Can you work these out from the model? Positions are in its coordinate system, mm. Face numbers are marked on the shaded views. A direction names the side the tool comes from. Give positions to 0.01 mm unless a question says otherwise; leave off trailing zeros. Order: outer loops, then holes, each group sorted by start corner. A loop starts at its lowest first (then second) coordinate and runs counter-clockwise, first axis right, second up. Notation, with made-up numbers: (83, 50) - (116, 50) arc R17 cw to (116, 76) - close; hole circle Ø5 at (2.25, 39.25). An arc over 180 degrees is marked (long way). Use one line per item in the form item = value. Start each with the question number.
1) Suppose I cut it at A-A, the plane y = 36. Write out the boundary of the cut face in (x, z), and give its area (3 significant figures).
2) Suppose I cut it at D-D, the plane y = 0. Write out the boundary of the cut face in (x, z), and give its area (3 significant figures).
3) Please list where these lines run through material, in increasing order: probe 1 along Z at (x, y) = (9.4, 0); probe 2 along Z at (x, y) = (-62, -10); probe 3 along X at (y, z) = (-7, 68.5).
4) Suppose I cut it at B-B, the plane x = -11. Write out the boundary of the cut face in (y, z).
5) Suppose I cut it at C-C, the plane z = 32. Write out the boundary of the cut face in (x, y), and give its area (3 significant figures).
6) Which directions (+Z, -Z, +X, -X, +Y, -Y) give clear straight access to the entire face, cutting with the end or side of a thin tool? Please do the marked faces 1, 2, 3, 4 and 5.
7) For pin 1 (12 mm diameter, centred on y = 65.5, z = 15.5, fed in from +X); pin 2 (9 mm diameter, centred on y = -6.5, z = 113.5, fed in from -X); pin 3 (1 mm diameter, centred on y = 22, z = 72, fed in from +X); pin 4 (12 mm diameter, centred on x = -35.5, y = 19, fed in from +Z), each with a flat end and sliding along its axis, tell me the tip position at first contact or that it passes through.
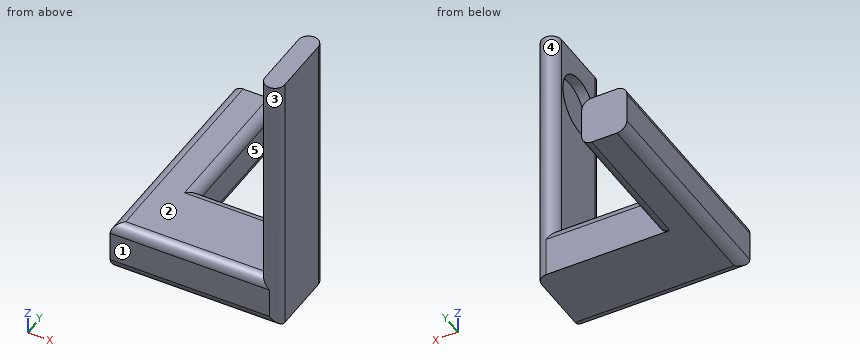
```python
from build123d import *

# Parameters (mm, degrees)
F0_W         = 70
F0_H         = 40
F0_W_2       = 15
F1_DEPTH     = 25
F2_W         = 10
F2_H         = 40
F3_DEPTH     = 110
F4_W         = 22.7000065148
F4_H         = 25
F5_DEPTH     = 70
F6_R         = 14.75
F7_DEPTH     = 5
F8_T1_DEPTH  = 87.5
F8_T3_DEPTH  = 52.2999934852
F8_T5_DEPTH  = 82.5
F8_T7_DEPTH  = 135
F8_T9_DEPTH  = 110
F8_T11_DEPTH = 160
F8_T13_DEPTH = 122.5
F8_T19_DEPTH = 100
F8_T23_DEPTH = 135
F8_T30_DEPTH = 64.7999934852
F8_T34_DEPTH = 135
F8_T41_DEPTH = 64.7999934852
F8_T45_DEPTH = 95


# Not quite as in the source:
# - a fillet or chamfer that OpenCascade refuses, or shapes differently, is made with other operations: its cross-section is extruded or revolved along the edge and cut away or added


with BuildPart() as f1:
    # F0 (on Top) → F1 (new body)
    with BuildSketch(Plane.XY):
        with Locations((-33.8003174961, 0.9457613719)):
            Rectangle(F0_W, F0_H)
        with Locations((8.6996825039, 0.9457613719)):
            Rectangle(F0_W_2, F0_H)
    extrude(amount=F1_DEPTH)

    # F2 (on face) → F3 (join)
    with BuildSketch(Plane.XY.offset(25)):
        with Locations((11.1996825039, 0.9457613719)):
            Rectangle(F2_W, F2_H)
    extrude(amount=F3_DEPTH)

    # F4 (on face) → F5 (join)
    with BuildSketch(Plane(origin=(0, 20.9457613719, 0), x_dir=(-1, 0, 0), z_dir=(0, 1, 0))):
        with Locations((57.4503142387, 12.5)):
            Rectangle(F4_W, F4_H)
    extrude(amount=F5_DEPTH)

    # F6 (on face) → F7 (cut)
    with BuildSketch(Plane(origin=(6.1996825039, 0, 0), x_dir=(0, -1, 0), z_dir=(-1, 0, 0))):
        with Locations((0, 108.7849736214)):
            Circle(F6_R)
    extrude(amount=-F7_DEPTH, mode=Mode.SUBTRACT)

    # F8: fillet of radius 5 on 11 edges, made by hand

    # F8_s2 → F8_t1 (cut)
    with BuildSketch(Plane.YZ.offset(-81.3003174961)):
        with BuildLine():
            ThreePointArc((-19.0542386281, 20), (-17.589772534, 23.5355339059), (-14.0542386281, 25))
            Line((-14.0542386281, 25), (-19.0542386281, 25))
            Line((-19.0542386281, 25), (-19.0542386281, 20))
        make_face()
    extrude(amount=F8_T1_DEPTH, mode=Mode.SUBTRACT)

    # F8_s4 → F8_t3 (cut)
    with BuildSketch(Plane.YZ.offset(-46.1003109813)):
        with BuildLine():
            ThreePointArc((15.9457613719, 25), (19.4812952778, 23.5355339059), (20.9457613719, 20))
            Line((20.9457613719, 20), (20.9457613719, 25))
            Line((20.9457613719, 25), (15.9457613719, 25))
        make_face()
    extrude(amount=F8_T3_DEPTH, mode=Mode.SUBTRACT)

    # F8_s6 → F8_t5 (cut)
    with BuildSketch(Plane.XZ.offset(-103.4457613719)):
        with BuildLine():
            ThreePointArc((-51.1003109813, 25), (-47.5647770753, 23.5355339059), (-46.1003109813, 20))
            Line((-46.1003109813, 20), (-46.1003109813, 25))
            Line((-46.1003109813, 25), (-51.1003109813, 25))
        make_face()
        with BuildLine():
            ThreePointArc((-51.1003109813, 0), (-47.5647770753, 1.4644660941), (-46.1003109813, 5))
            Line((-46.1003109813, 5), (-46.1003109813, 0))
            Line((-46.1003109813, 0), (-51.1003109813, 0))
        make_face()
    extrude(amount=F8_T5_DEPTH, mode=Mode.SUBTRACT)

    # F8_s8 → F8_t7 (cut)
    with BuildSketch(Plane.XZ.offset(-103.4457613719)):
        with BuildLine():
            ThreePointArc((-68.8003174961, 20), (-67.335851402, 23.5355339059), (-63.8003174961, 25))
            Line((-63.8003174961, 25), (-68.8003174961, 25))
            Line((-68.8003174961, 25), (-68.8003174961, 20))
        make_face()
        with BuildLine():
            ThreePointArc((-68.8003174961, 5), (-67.335851402, 1.4644660941), (-63.8003174961, 0))
            Line((-63.8003174961, 0), (-68.8003174961, 0))
            Line((-68.8003174961, 0), (-68.8003174961, 5))
        make_face()
    extrude(amount=F8_T7_DEPTH, mode=Mode.SUBTRACT)

    # F8_s10 → F8_t9 (cut)
    with BuildSketch(Plane.YZ.offset(-81.3003174961)):
        with BuildLine():
            ThreePointArc((-19.0542386281, 5), (-17.589772534, 1.4644660941), (-14.0542386281, 0))
            Line((-14.0542386281, 0), (-19.0542386281, 0))
            Line((-19.0542386281, 0), (-19.0542386281, 5))
        make_face()
    extrude(amount=F8_T9_DEPTH, mode=Mode.SUBTRACT)

    # F8_s12 → F8_t11 (cut)
    with BuildSketch(Plane.XY.offset(-12.5)):
        with BuildLine():
            ThreePointArc((11.1996825039, -19.0542386281), (14.7352164099, -17.589772534), (16.1996825039, -14.0542386281))
            Line((16.1996825039, -14.0542386281), (16.1996825039, -19.0542386281))
            Line((16.1996825039, -19.0542386281), (11.1996825039, -19.0542386281))
        make_face()
        with BuildLine():
            ThreePointArc((16.1996825039, 15.9457613719), (14.7352164099, 19.4812952778), (11.1996825039, 20.9457613719))
            Line((11.1996825039, 20.9457613719), (16.1996825039, 20.9457613719))
            Line((16.1996825039, 20.9457613719), (16.1996825039, 15.9457613719))
        make_face()
    extrude(amount=F8_T11_DEPTH, mode=Mode.SUBTRACT)

    # F8_s14 → F8_t13 (cut)
    with BuildSketch(Plane.XY.offset(25)):
        with BuildLine():
            ThreePointArc((11.1996825039, -19.0542386281), (7.664148598, -17.589772534), (6.1996825039, -14.0542386281))
            Line((6.1996825039, -14.0542386281), (6.1996825039, -19.0542386281))
            Line((6.1996825039, -19.0542386281), (11.1996825039, -19.0542386281))
        make_face()
        with BuildLine():
            ThreePointArc((6.1996825039, 15.9457613719), (7.664148598, 19.4812952778), (11.1996825039, 20.9457613719))
            Line((11.1996825039, 20.9457613719), (6.1996825039, 20.9457613719))
            Line((6.1996825039, 20.9457613719), (6.1996825039, 15.9457613719))
        make_face()
    extrude(amount=F8_T13_DEPTH, mode=Mode.SUBTRACT)


with BuildPart() as f8_tool17:
    # F8_s18 → F8_t19 (new body)
    with BuildSketch(Plane.YZ.offset(-81.3003174961)):
        with BuildLine():
            ThreePointArc((-19.0542386281, 20), (-17.589772534, 23.5355339059), (-14.0542386281, 25))
            Line((-14.0542386281, 25), (-19.0542386281, 25))
            Line((-19.0542386281, 25), (-19.0542386281, 20))
        make_face()
    extrude(amount=F8_T19_DEPTH)

    split(bisect_by=Plane.YZ.offset(6.1996825039), keep=Keep.TOP)


with BuildPart() as f8_tool21:
    # F8_s22 → F8_t23 (new body)
    with BuildSketch(Plane.XY.offset(12.5)):
        with BuildLine():
            ThreePointArc((11.1996825039, -19.0542386281), (7.664148598, -17.589772534), (6.1996825039, -14.0542386281))
            Line((6.1996825039, -14.0542386281), (6.1996825039, -19.0542386281))
            Line((6.1996825039, -19.0542386281), (11.1996825039, -19.0542386281))
        make_face()
    extrude(amount=F8_T23_DEPTH)

    split(bisect_by=Plane.XY.offset(25), keep=Keep.BOTTOM)


with BuildPart() as f8_tool17_1:
    add(f8_tool17.part)

    # F8_t25: intersect F8_tool21
    add(f8_tool21.part, mode=Mode.INTERSECT)


with BuildPart() as f1_1:
    add(f1.part)

    # F8_t15: cut F8_tool17
    add(f8_tool17_1.part, mode=Mode.SUBTRACT)


with BuildPart() as f8_tool28:
    # F8_s29 → F8_t30 (new body)
    with BuildSketch(Plane.YZ.offset(18.6996825039)):
        with BuildLine():
            ThreePointArc((15.9457613719, 25), (19.4812952778, 23.5355339059), (20.9457613719, 20))
            Line((20.9457613719, 20), (20.9457613719, 25))
            Line((20.9457613719, 25), (15.9457613719, 25))
        make_face()
    extrude(amount=-F8_T30_DEPTH)

    split(bisect_by=Plane.YZ.offset(6.1996825039), keep=Keep.TOP)


with BuildPart() as f8_tool32:
    # F8_s33 → F8_t34 (new body)
    with BuildSketch(Plane.XY.offset(12.5)):
        with BuildLine():
            ThreePointArc((6.1996825039, 15.9457613719), (7.664148598, 19.4812952778), (11.1996825039, 20.9457613719))
            Line((11.1996825039, 20.9457613719), (6.1996825039, 20.9457613719))
            Line((6.1996825039, 20.9457613719), (6.1996825039, 15.9457613719))
        make_face()
    extrude(amount=F8_T34_DEPTH)

    split(bisect_by=Plane.XY.offset(25), keep=Keep.BOTTOM)


with BuildPart() as f8_tool28_1:
    add(f8_tool28.part)

    # F8_t36: intersect F8_tool32
    add(f8_tool32.part, mode=Mode.INTERSECT)


with BuildPart() as f1_2:
    add(f1_1.part)

    # F8_t26: cut F8_tool28
    add(f8_tool28_1.part, mode=Mode.SUBTRACT)


with BuildPart() as f8_tool39:
    # F8_s40 → F8_t41 (new body)
    with BuildSketch(Plane.YZ.offset(6.1996825039)):
        with BuildLine():
            ThreePointArc((15.9457613719, 25), (19.4812952778, 23.5355339059), (20.9457613719, 20))
            Line((20.9457613719, 20), (20.9457613719, 25))
            Line((20.9457613719, 25), (15.9457613719, 25))
        make_face()
    extrude(amount=-F8_T41_DEPTH)

    split(bisect_by=Plane.YZ.offset(-46.1003109813), keep=Keep.BOTTOM)


with BuildPart() as f8_tool43:
    # F8_s44 → F8_t45 (new body)
    with BuildSketch(Plane.XZ.offset(-8.4457613719)):
        with BuildLine():
            ThreePointArc((-51.1003109813, 25), (-47.5647770753, 23.5355339059), (-46.1003109813, 20))
            Line((-46.1003109813, 20), (-46.1003109813, 25))
            Line((-46.1003109813, 25), (-51.1003109813, 25))
        make_face()
    extrude(amount=-F8_T45_DEPTH)

    split(bisect_by=Plane.XZ.offset(-20.9457613719), keep=Keep.TOP)


with BuildPart() as f8_tool39_1:
    add(f8_tool39.part)

    # F8_t47: intersect F8_tool43
    add(f8_tool43.part, mode=Mode.INTERSECT)


with BuildPart() as f1_3:
    add(f1_2.part)

    # F8_t37: cut F8_tool39
    add(f8_tool39_1.part, mode=Mode.SUBTRACT)


solid = f1_3.part
```
Result sheet:
q1.outline = (-68.8, 5) arc R5 ccw to (-63.8, 0) - (-51.1, 0) arc R5 ccw to (-46.1, 5) - (-46.1, 20) arc R5 ccw to (-51.1, 25) - (-63.8, 25) arc R5 ccw to (-68.8, 20) - close
q1.area = 546 mm²
q2.outline = (-68.8, 5) arc R5 ccw to (-63.8, 0) - (16.2, 0) - (16.2, 135) - (6.2, 135) - (6.2, 123.53) - (11.2, 123.53) - (11.2, 94.03) - (6.2, 94.03) - (6.2, 25) - (-63.8, 25) arc R5 ccw to (-68.8, 20) - close
q2.area = 3,070 mm²
q3.probe_1 = 0 to 94.03, 123.53 to 135
q3.probe_2 = 0 to 25
q3.probe_3 = 6.2 to 16.2
q4.outline = (-19.05, 5) arc R5 ccw to (-14.05, 0) - (20.95, 0) - (20.95, 20) arc R5 ccw to (15.95, 25) - (-14.05, 25) arc R5 ccw to (-19.05, 20) - close
q5.outline = (6.2, -14.05) arc R5 ccw to (16.2, -14.05) - (16.2, 15.95) arc R5 ccw to (6.2, 15.95) - close
q5.area = 379 mm²
q6.face_1 = +Z, -Z, +X, -X, -Y
q6.face_2 = +Z, -X, +Y, -Y
q6.face_3 = +Z, -Y
q6.face_4 = +Z, +Y
q6.face_5 = +Z, -Z, +X, +Y
q7.pin_1 = -46.1
q7.pin_2 = 11.2
q7.pin_3 = through
q7.pin_4 = 25
